Verification items for the finished model (mm, model axes). Face numbers are marked on the shaded views. A direction names the side the tool comes from. Round coordinates to 2 decimals unless told otherwise and drop trailing zeros. Write each loop counter-clockwise with the first axis right and the second up, starting at its lowest first coordinate (ties: lowest second). Pieces come first, ordered by that corner, then holes. Notation, with made-up numbers: M -39.75,6 L -16.75,6 A28 ccw -16.75,26 Z; hole C -19.75,68.5 d6. An arc over 180 degrees is marked long. One line per question, with ' | ' between items.
from build123d import *

# Parameters (mm, degrees)
SKETCH1_R           = 6.5
BOSS_EXTRUDE1_DEPTH = 20
SKETCH2_R           = 11.5
CUT_EXTRUDE1_DEPTH  = 21
BOSS_EXTRUDE2_DEPTH = 25
SKETCH3_R           = 72.5
SKETCH3_R_2         = 52.5
CUT_EXTRUDE2_DEPTH  = 3
FILLET2_R           = 12


with BuildPart() as part:
    # Sketch1 → Boss-Extrude1 (new body)
    with BuildSketch(Plane(origin=(0, 0, 0), x_dir=(1, 0, 0), z_dir=(0, 1, 0))):
        with BuildLine():
            Line((-89.148145657, 58.529523872), (-78.104184034, 17.312897978))
            ThreePointArc((-78.104184034, 17.312897978), (-80, 0), (-78.104184034, -17.312897978))
            Line((-78.104184034, -17.312897978), (-89.148145657, -58.529523872))
            ThreePointArc((-89.148145657, -58.529523872), (-82.67766953, -82.67766953), (-58.529523872, -89.148145657))
            Line((-58.529523872, -89.148145657), (-17.312897978, -78.104184034))
            ThreePointArc((-17.312897978, -78.104184034), (0, -80), (17.312897978, -78.104184034))
            Line((17.312897978, -78.104184034), (58.529523872, -89.148145657))
            ThreePointArc((58.529523872, -89.148145657), (82.67766953, -82.67766953), (89.148145657, -58.529523872))
            Line((89.148145657, -58.529523872), (78.104184034, -17.312897978))
            ThreePointArc((78.104184034, -17.312897978), (80, 0), (78.104184034, 17.312897978))
            Line((78.104184034, 17.312897978), (89.148145657, 58.529523872))
            ThreePointArc((89.148145657, 58.529523872), (82.67766953, 82.67766953), (58.529523872, 89.148145657))
            Line((58.529523872, 89.148145657), (17.312897978, 78.104184034))
            ThreePointArc((17.312897978, 78.104184034), (0, 80), (-17.312897978, 78.104184034))
            Line((-17.312897978, 78.104184034), (-58.529523872, 89.148145657))
            ThreePointArc((-58.529523872, 89.148145657), (-82.67766953, 82.67766953), (-89.148145657, 58.529523872))
        make_face()
        with Locations((-65, 65)):
            Circle(SKETCH1_R, mode=Mode.SUBTRACT)
        with Locations((65, 65)):
            Circle(SKETCH1_R, mode=Mode.SUBTRACT)
        with Locations((65, -65)):
            Circle(SKETCH1_R, mode=Mode.SUBTRACT)
        with Locations((-65, -65)):
            Circle(SKETCH1_R, mode=Mode.SUBTRACT)
    extrude(amount=BOSS_EXTRUDE1_DEPTH)

    # Sketch2 → Cut-Extrude1 (cut, through all)
    with BuildSketch(Plane(origin=(0, 20, 0), x_dir=(1, 0, 0), z_dir=(0, 1, 0))):
        with Locations((-22, -22)):
            Circle(SKETCH2_R)
        with Locations((-22, 22)):
            Circle(SKETCH2_R)
        with Locations((22, 22)):
            Circle(SKETCH2_R)
        with Locations((22, -22)):
            Circle(SKETCH2_R)
    extrude(amount=-CUT_EXTRUDE1_DEPTH, mode=Mode.SUBTRACT)

    # Sketch2<3> → Boss-Extrude2 (add)
    with BuildSketch(Plane(origin=(0, 20, 0), x_dir=(1, 0, 0), z_dir=(0, 1, 0))):
        with BuildLine():
            Line((-35, -50), (35, -50))
            ThreePointArc((35, -50), (45.606601718, -45.606601718), (50, -35))
            Line((50, -35), (50, 35))
            ThreePointArc((50, 35), (45.606601718, 45.606601718), (35, 50))
            Line((35, 50), (-35, 50))
            ThreePointArc((-35, 50), (-45.606601718, 45.606601718), (-50, 35))
            Line((-50, 35), (-50, -35))
            ThreePointArc((-50, -35), (-45.606601718, -45.606601718), (-35, -50))
        make_face()
        with BuildLine():
            Line((-44, -35), (-44, 35))
            ThreePointArc((-44, 35), (-41.363961031, 41.363961031), (-35, 44))
            Line((-35, 44), (35, 44))
            ThreePointArc((35, 44), (41.363961031, 41.363961031), (44, 35))
            Line((44, 35), (44, -35))
            ThreePointArc((44, -35), (41.363961031, -41.363961031), (35, -44))
            Line((35, -44), (-35, -44))
            ThreePointArc((-35, -44), (-41.363961031, -41.363961031), (-44, -35))
        make_face(mode=Mode.SUBTRACT)
    extrude(amount=BOSS_EXTRUDE2_DEPTH)

    # Sketch3 → Cut-Extrude2 (cut)
    with BuildSketch(Plane.XZ):
        Circle(SKETCH3_R)
        Circle(SKETCH3_R_2, mode=Mode.SUBTRACT)
    extrude(amount=-CUT_EXTRUDE2_DEPTH, mode=Mode.SUBTRACT)

    # Fillet2
    fillet2_edges = [part.edges().sort_by_distance(p)[0] for p in [
        (-17.312897978, 10, -78.104184034),
        (17.312897978, 10, -78.104184034),
        (78.104184034, 10, -17.312897978),
        (78.104184034, 10, 17.312897978),
        (17.312897978, 10, 78.104184034),
        (-17.312897978, 10, 78.104184034),
        (-78.104184034, 10, 17.312897978),
        (-78.104184034, 10, -17.312897978),
    ]]
    fillet(fillet2_edges, radius=FILLET2_R)


solid = part.part
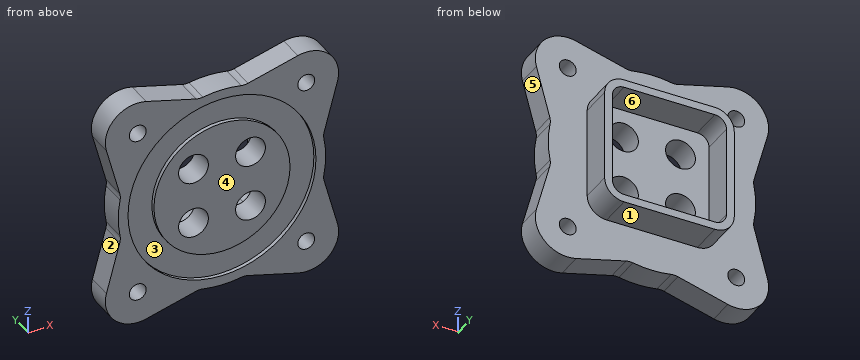
1. Thickness scan on line 1 (Z direction, x = 65, y = 4); line 2 (X direction, y = 4.5, z = -22). Record the ranges inside material, lowest first.
Results:
line 1: z = -90 to -71.5, -58.5 to 58.5, 71.5 to 90 | line 2: x = -79.36 to -33.5, -10.5 to 10.5, 33.5 to 79.36
2. Go/stop test with flat-tipped pins: P1, Ø15, axis at x = -65, z = 65, coming from the +Y side; P2, Ø1, axis at y = 18.5, z = -27, coming from the -X side; P3, Ø3, axis at x = 45, z = 51.5, coming from the -Y side. Record where each tip stops, or that it passes through.
Results:
P1: stops at y = 20 | P2: stops at x = -80.83 | P3: stops at y = 3
3. Section check A-A, the plane y = 13. Count the separate pieces of the cut face and the enclosed holes in it, then the cut area to 3 significant figures.
Results:
separate pieces: 1 | enclosed holes: 8 | area: 26,100 mm2
4. Section check B-B, the plane x = 0. Record the cut outline in (y, z), then the cut area to 3 significant figures.
Results:
outline: M 0,-80 L 20,-80 L 20,-50 L 45,-50 L 45,-44 L 20,-44 L 20,44 L 45,44 L 45,50 L 20,50 L 20,80 L 0,80 L 0,72.5 L 3,72.5 L 3,52.5 L 0,52.5 L 0,-52.5 L 3,-52.5 L 3,-72.5 L 0,-72.5 Z | area: 3,380 mm2
5. Section check D-D, the plane y = 26.5. Record the cut outline in (x, z), then the cut area to 3 significant figures.
Results:
outline: M -50,-35 A15 ccw -35,-50 L 35,-50 A15 ccw 50,-35 L 50,35 A15 ccw 35,50 L -35,50 A15 ccw -50,35 Z; hole M -44,-35 A9 ccw -35,-44 L 35,-44 A9 ccw 44,-35 L 44,35 A9 ccw 35,44 L -35,44 A9 ccw -44,35 Z | area: 2,130 mm2
6. Tool access check on the marked faces 1, 2 and 3. Record the directions out of +Z, -Z, +X, -X, +Y, -Y that give a thin tool (end or side, any length) a straight path to the whole face; none if there is none.
Results:
face 1: -Z, +X, -X, +Y | face 2: -X, +Y, -Y | face 3: -Y
7. Section check C-C, the plane z = 65. Record the cut outline in (x, y), then the cut area to 3 significant figures.
Results:
outline: M -90,0 L -71.5,0 L -71.5,20 L -90,20 Z; M -58.5,0 L -32.11,0 L -32.11,3 L 32.11,3 L 32.11,0 L 58.5,0 L 58.5,20 L -58.5,20 Z; M 71.5,0 L 90,0 L 90,20 L 71.5,20 Z | area: 2,890 mm2
8. Mould release check, pull along X, two halves, no side actions. Record for the marked faces 4, 5 and 6: pulls with the +X half, pulls with the -X half, needs draft (parallel to the pull), parting line crosses it, or undercut.
Results:
face 4: needs draft | face 5: pulls with the +X half | face 6: undercut
